Source: CAD feature listing. Evaluate the final solid. Frame: model axes, mm. Face numbers are marked on the shaded views. A direction names the side the tool comes from. Give positions to 0.01 mm unless a question says otherwise; leave off trailing zeros. Order: outer loops, then holes, each group sorted by start corner. A loop starts at its lowest first (then second) coordinate and runs counter-clockwise, first axis right, second up. Notation, with made-up numbers: M 71,87 L 85,87 A27 ccw 85,123 Z; hole C -10.5,-12.75 d8. An arc over 180 degrees is marked long. Answer in a Markdown table with one row per item. Add a question column.
(1) Section query C-C, the plane z = 7.5. Count the separate pieces of the cut face and the enclosed holes in it, plus the area to 3 significant figures.
(2) Set-up query: the marked faces 4 and 5. Return all of +Z, -Z, +X, -X, +Y, -Y with unobstructed straight access to the full face (end or side cutting, diameter ignored); none if empty.
(3) Section query D-D, the plane z = 12.25. Return loops of the section in (x, y).
(4) Section query B-B, the plane x = -12.5. Return loops of the section in (y, z), plus the area to 3 significant figures.
(5) Mould query, pull axis X, two halves, no side actions, for the marked faces 1, 2 and 3. Classes: pulls with the +X half, pulls with the -X half, needs draft (parallel to the pull), parting line crosses it, or undercut.
(6) Material intervals for line 1 along X through (y, z) = (1, 10.25); line 2 along Z through (x, y) = (9, 17.6); line 3 along X through (y, z) = (15.25, 6.5), sorted ascending.
(7) Section query A-A, the plane x = 9. Return loops of the section in (y, z), plus the area to 3 significant figures.
(8) Pin query (flat end, axial travel): P1, Ø6.5, axis at x = 9, z = 7.5, coming from the -Y side; P2, Ø2, axis at y = 17.5, z = 9, coming from the +X side. Return the tip coordinate at first contact, or that it passes through.
from build123d import *

# Parameters (mm, degrees)
BOSS_EXTRU_1_DEPTH      = 15
CHANFREIN1_SIZE         = 5
CHANFREIN2_SIZE         = 7
TROU_TARAUD_M6X1_01_D   = 5
TROU_TARAUD_M3X0_51_D   = 2.5
CHANFREIN6_SIZE         = 0.5
CHANFREIN10_SIZE        = 0.5
CHANFREIN10_EDGE_2_SIZE = 0.5
CHANFREIN10_EDGE_3_SIZE = 0.5
CHANFREIN10_EDGE_4_SIZE = 0.5


with BuildPart() as part:
    # Esquisse1 → Boss.-Extru.1 (new body)
    with BuildSketch(Plane.XY):
        Polygon((-30, 0), (-39, 0), (-39, 20), (39, 20), (39, 0), (30, 0), (30, 15), (-30, 15), align=None)
    extrude(amount=BOSS_EXTRU_1_DEPTH)

    # Chanfrein1
    chanfrein1_edges = [part.edges().sort_by_distance(p)[0] for p in [
        (30, 15, 7.5),
        (-30, 15, 7.5),
    ]]
    chamfer(chanfrein1_edges, length=CHANFREIN1_SIZE)

    # Chanfrein2
    chanfrein2_edges = [part.edges().sort_by_distance(p)[0] for p in [
        (-39, 20, 7.5),
        (39, 20, 7.5),
    ]]
    chamfer(chanfrein2_edges, length=CHANFREIN2_SIZE)

    # Trou taraudé M6x1.01 (through all)
    with Locations(Plane(origin=(0, 20, 0), x_dir=(1, 0, 0), z_dir=(0, 1, 0))):
        with Locations((9, -7.5), (-9, -7.5)):
            Hole(TROU_TARAUD_M6X1_01_D / 2)

    # Trou taraudé M3x0.51 (through all)
    with Locations(Plane(origin=(0, 0, 0), x_dir=(-1, 0, 0), z_dir=(0, -1, 0))):
        with Locations((-34.5, -7.5), (34.5, -7.5)):
            Hole(TROU_TARAUD_M3X0_51_D / 2)

    # Chanfrein6
    chanfrein6_edges = [part.edges().sort_by_distance(p)[0] for p in [
        (34.5, 0, 0),
        (-30, 5, 0),
        (-30, 0, 7.5),
        (-39, 0, 7.5),
        (39, 0, 7.5),
        (30, 0, 7.5),
        (34.5, 0, 15),
        (39, 6.5, 15),
        (0, 15, 0),
        (0, 15, 15),
        (30, 5, 0),
        (30, 5, 15),
        (-27.5, 12.5, 0),
        (-27.5, 12.5, 15),
        (27.5, 12.5, 0),
        (27.5, 12.5, 15),
        (-34.5, 0, 15),
        (0, 20, 0),
        (0, 20, 15),
        (-39, 6.5, 0),
        (-35.5, 16.5, 0),
        (35.5, 16.5, 0),
        (-39, 6.5, 15),
        (-35.5, 16.5, 15),
        (35.5, 16.5, 15),
        (-30, 5, 15),
        (-34.5, 0, 0),
        (39, 6.5, 0),
    ]]
    chamfer(chanfrein6_edges, length=CHANFREIN6_SIZE)

    # Chanfrein10
    chanfrein10_edges = [part.edges().sort_by_distance(p)[0] for p in [
        (39, 13, 7.5),
    ]]
    chamfer(chanfrein10_edges, length=CHANFREIN10_SIZE)

    # Chanfrein10 edge 2
    chanfrein10_edge_2_edges = [part.edges().sort_by_distance(p)[0] for p in [
        (32, 20, 7.5),
    ]]
    chamfer(chanfrein10_edge_2_edges, length=CHANFREIN10_EDGE_2_SIZE)

    # Chanfrein10 edge 3
    chanfrein10_edge_3_edges = [part.edges().sort_by_distance(p)[0] for p in [
        (-32, 20, 7.5),
    ]]
    chamfer(chanfrein10_edge_3_edges, length=CHANFREIN10_EDGE_3_SIZE)

    # Chanfrein10 edge 4
    chanfrein10_edge_4_edges = [part.edges().sort_by_distance(p)[0] for p in [
        (-39, 13, 7.5),
    ]]
    chamfer(chanfrein10_edge_4_edges, length=CHANFREIN10_EDGE_4_SIZE)


solid = part.part
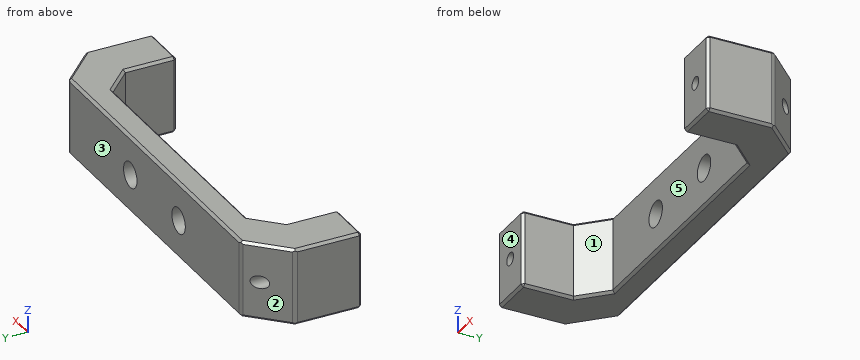
Values follow:
| question | item | result |
|---|---|---|
| 1 | separate pieces | 5 |
| 1 | enclosed holes | 0 |
| 1 | area | 498 mm² |
| 2 | face 4 | +Z, -Z, +X, -X, -Y |
| 2 | face 5 | +Z, -Z, -Y |
| 3 | outline | M -39,0.5 L -38.5,0 L -30.5,0 L -30,0.5 L -30,10 L -25,15 L 25,15 L 30,10 L 30,0.5 L 30.5,0 L 38.5,0 L 39,0.5 L 39,12.5 L 38.65,13.35 L 32.35,19.65 L 31.5,20 L -31.5,20 L -32.35,19.65 L -38.65,13.35 L -39,12.5 Z |
| 4 | outline | M 15,0.5 L 15.5,0 L 19.5,0 L 20,0.5 L 20,14.5 L 19.5,15 L 15.5,15 L 15,14.5 Z |
| 4 | area | 74.5 mm² |
| 5 | face 1 | undercut |
| 5 | face 2 | pulls with the -X half |
| 5 | face 3 | needs draft |
| 6 | line 1 | x = -39 to -30, 30 to 39 |
| 6 | line 2 | z = 0 to 5, 10 to 15 |
| 6 | line 3 | x = -36.75 to -35.25, -33.75 to -11.29, -6.71 to 6.71, 11.29 to 33.75, 35.25 to 36.75 |
| 7 | outline | M 15,0.5 L 15.5,0 L 19.5,0 L 20,0.5 L 20,5 L 15,5 Z; M 15,10 L 20,10 L 20,14.5 L 19.5,15 L 15.5,15 L 15,14.5 Z |
| 7 | area | 49.5 mm² |
| 8 | P1 | stops at y = 15 |
| 8 | P2 | stops at x = 35.5 |
